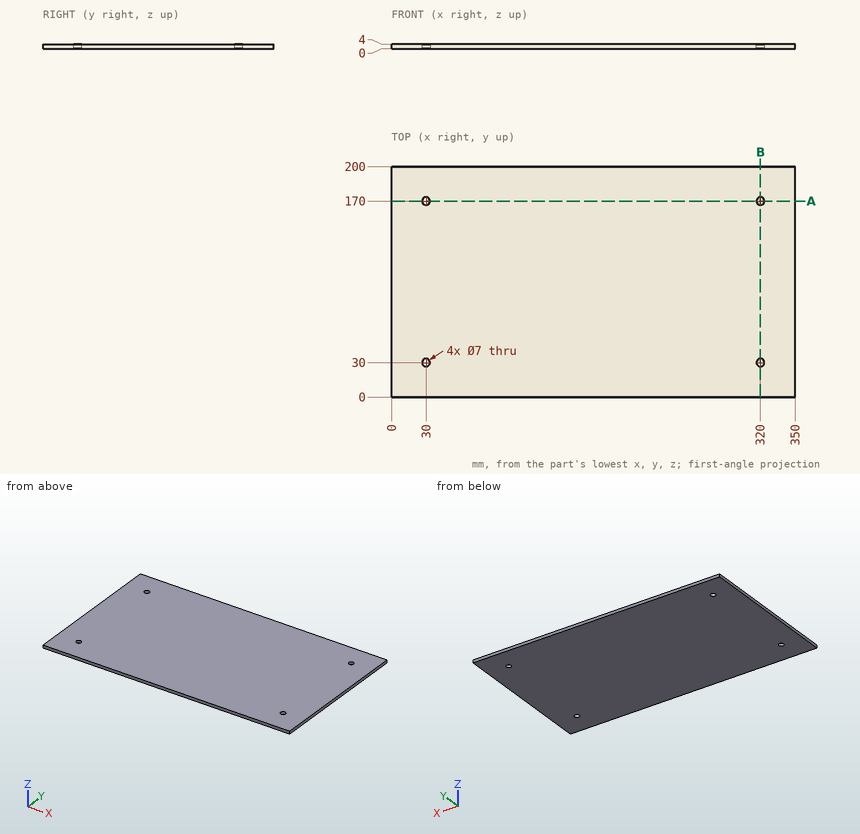
Here's the drawing with two shaded views (mm, measured from the low corner). I have some questions. Give positions to 0.01 mm unless a question says otherwise; leave off trailing zeros. Write each loop counter-clockwise with the first axis right and the second up, starting at its lowest first coordinate (ties: lowest second). Pieces come first, ordered by that corner, then holes. Notation, with made-up numbers: (63.25, -19) -> (73.25, -19) arc R9 cw to (73.25, -8) -> close; hole circle Ø9 at (76.25, 89). An arc over 180 degrees is marked (long way). One line per item, written item: value.
Q1. For P1, Ø4, axis at x = 320, y = 30, coming from the -Z side, with a flat end and sliding along its axis, tell me the tip position at first contact or that it passes through.
Results found:
P1: passes through
Q2. Imagine slicing it at B-B on x = 320. Please give me the cut outline in (y, z).
Results found:
outline: (0, 0) -> (26.5, 0) -> (26.5, 4) -> (0, 4) -> close; (33.5, 0) -> (166.5, 0) -> (166.5, 4) -> (33.5, 4) -> close; (173.5, 0) -> (200, 0) -> (200, 4) -> (173.5, 4) -> close
Q3. Please list where these lines run through material, in increasing order: line 1 (X direction, y = 30, z = 1.4); line 2 (Y direction, x = 30, z = 2.35); line 3 (X direction, y = 168, z = 0.3). Write a range as [from, to].
Results found:
line 1: x = [0, 26.5], [33.5, 316.5], [323.5, 350]
line 2: y = [0, 26.5], [33.5, 166.5], [173.5, 200]
line 3: x = [0, 27.13], [32.87, 317.13], [322.87, 350]
Q4. Imagine slicing it at A-A on y = 170. Please give me the cut outline in (x, z).
Results found:
outline: (0, 0) -> (26.5, 0) -> (26.5, 4) -> (0, 4) -> close; (33.5, 0) -> (316.5, 0) -> (316.5, 4) -> (33.5, 4) -> close; (323.5, 0) -> (350, 0) -> (350, 4) -> (323.5, 4) -> close
